Can you work these out from the model? Positions are in its coordinate system, mm. Coordinates: 2 decimals unless noted, no trailing zeros. Order: outer loops, then holes, each group sorted by start corner. A loop starts at its lowest first (then second) coordinate and runs counter-clockwise, first axis right, second up. Notation, with made-up numbers: (88.5, 21) -> (109.5, 21) arc R20 cw to (109.5, 51) -> close; hole circle Ø2 at (38, 56). An arc over 180 degrees is marked (long way). Answer as a JSON object with one key per item and string values. Group by question number.
(1) I want a section at B-B, the plane y = 8. List the corners of the cut face in (x, z) for me.
(2) If we mould it in two halves opening along X, with no side actions, what happens to faces 1 (the cylindrical face through (3.09, 7.3, 2.96)), 2 (the flat face through (52, 10, 3)), 3 (the flat face through (26, 0, 3))? For each: pulls with the +X half, pulls with the -X half, needs draft (parallel to the pull), parting line crosses it, or undercut.
(3) I need wall thicknesses on line 1 (Y direction, x = 48, z = 3); line 2 (Y direction, x = 26, z = 1.75); line 3 (X direction, y = 20, z = 4.3). Which ranges of each line are inside material? Lowest first, please.
(4) I want a section at C-C, the plane z = 3.2. List the corners of the cut face in (x, y) for me.
(5) For pin 1 (3.5 mm diameter, centred on x = 4, y = 8, fed in from -Z); pin 2 (2.5 mm diameter, centred on x = 26, y = 21, fed in from -Z), each with a flat end and sliding along its axis, tell me the tip position at first contact or that it passes through.
(6) I want a section at A-A, the plane x = 26. List the corners of the cut face in (y, z) for me.
from build123d import *

# Parameters (mm, degrees)
SKETCH1_R           = 1.5
SKETCH1_R_2         = 1.15
BOSS_EXTRUDE1_DEPTH = 6


with BuildPart() as part:
    # Sketch1 → Boss-Extrude1 (new body)
    with BuildSketch(Plane.XY):
        with BuildLine():
            Line((0, 0), (52, 0))
            Line((52, 0), (52, 21))
            ThreePointArc((52, 21), (50.828427125, 23.828427125), (48, 25))
            Line((48, 25), (4, 25))
            ThreePointArc((4, 25), (1.171572875, 23.828427125), (0, 21))
            Line((0, 21), (0, 0))
        make_face()
        with Locations((4, 21)):
            Circle(SKETCH1_R, mode=Mode.SUBTRACT)
        with Locations((48, 21)):
            Circle(SKETCH1_R, mode=Mode.SUBTRACT)
        with Locations((4, 8)):
            Circle(SKETCH1_R_2, mode=Mode.SUBTRACT)
        with Locations((48, 8)):
            Circle(SKETCH1_R_2, mode=Mode.SUBTRACT)
        with Locations((26, 21)):
            Circle(SKETCH1_R, mode=Mode.SUBTRACT)
    extrude(amount=BOSS_EXTRUDE1_DEPTH)


solid = part.part
Computed values:
{
 "1": {"outline": "(0, 0) -> (2.85, 0) -> (2.85, 6) -> (0, 6) -> close; (5.15, 0) -> (46.85, 0) -> (46.85, 6) -> (5.15, 6) -> close; (49.15, 0) -> (52, 0) -> (52, 6) -> (49.15, 6) -> close"},
 "2": {"face 1": "undercut", "face 2": "pulls with the +X half", "face 3": "needs draft"},
 "3": {"line 1": "y = 0 to 6.85, 9.15 to 19.5, 22.5 to 25", "line 2": "y = 0 to 19.5, 22.5 to 25", "line 3": "x = 0 to 2.88, 5.12 to 24.88, 27.12 to 46.88, 49.12 to 52"},
 "4": {"outline": "(0, 0) -> (52, 0) -> (52, 21) arc R4 ccw to (48, 25) -> (4, 25) arc R4 ccw to (0, 21) -> close; hole circle Ø3 at (4, 21); hole circle Ø2.3 at (4, 8); hole circle Ø3 at (26, 21); hole circle Ø3 at (48, 21); hole circle Ø2.3 at (48, 8)"},
 "5": {"pin 1": "stops at z = 0", "pin 2": "passes through"},
 "6": {"outline": "(0, 0) -> (19.5, 0) -> (19.5, 6) -> (0, 6) -> close; (22.5, 0) -> (25, 0) -> (25, 6) -> (22.5, 6) -> close"}
}
